Autodesk Inventor part; units mm, degrees
ref_plane "YZ Plane" through (0, 0, 0) normal (1, 0, 0) x (0, 1, 0)
ref_plane "XZ Plane" through (0, 0, 0) normal (0, 1, 0) x (-1, 0, 0)
ref_plane "XY Plane" through (0, 0, 0) normal (0, 0, 1) x (1, 0, 0)
sketch "スケッチ1" plane through (0, 0, 0) normal (0, 0, 1) x (1, 0, 0)
  line L0 (-6, 5) -> (6, 5)
  line L1 (6, 5) -> (6, -5)
  line L2 (6, -5) -> (-6, -5)
  line L3 (-6, -5) -> (-6, 5)
  point P0 (0, 0)
  point P1 (0, -5)
  point P2 (6, 0)
  dimension "d0" = 12
  dimension "d1" = 10
extrude "ギヤボックス" add sketch "スケッチ1" against normal blind 9
sketch "スケッチ2" plane through (0, 0, 0) normal (0, 0, 1) x (1, 0, 0)
  circle A0 centre (0, 0) radius 1.5
  line L0 (-1.118, 1) -> (1.118, 1)
  circle A1 centre (0, 0) radius 2
  dimension "d4" = 3
  dimension "d5" = 1
  dimension "d6" = 4
extrude "軸受け" add sketch "スケッチ2" along normal blind 0.7 contours A0 L0 | L0 A0 | A1
extrude "軸" add sketch "スケッチ2" along normal blind 10 contours A0 L0 picked at (0.0594, 0.1702)
sketch "スケッチ3" plane through (0, 0, -9) normal (0, 0, -1) x (-1, 0, 0)
  line L0 (6, 5) -> (-6, 5)
  line L1 (-6, -5) -> (6, -5)
  line L2 (-4, 5) -> (4, 5)
  line L3 (4, 5) -> (4, -5)
  line L4 (4, -5) -> (-4, -5)
  line L5 (-4, -5) -> (-4, 5)
  arc A0 (-4, 5) -> (-4, -5) centre (1.25, 0) ccw
  arc A1 (4, -5) -> (4, 5) centre (-1.25, 0) ccw
  line L6 (-6, 5) -> (-6, -5)
  line L7 (6, -5) -> (6, 5)
  line L8 (0, 7.0621) -> (0, -7.0621) construction
  line L9 (-6, 7.0625) -> (-6, -7.0625) construction
  line L10 (6, -7.0752) -> (6, 7.0489) construction
  point P0 (0, 0)
  point P1 (0, 5)
  point P2 (0, 0)
  point P3 (4, 5)
  point P4 (-4, -5)
  dimension "d11" = 8
  dimension "d15" = 12
extrude "モーター" add sketch "スケッチ3" along normal blind 15 contours L3 L1 L5 L0 | A1 L3 | L5 A0
sketch "スケッチ4" plane through (0, 0, -24) normal (0, 0, -1) x (-1, 0, 0)
  line L0 (-6.8, -5) -> (6.8, -5)
  line L1 (6.8, -5) -> (6.8, 5)
  line L2 (6.8, 5) -> (-6.8, 5)
  line L3 (-6.8, 5) -> (-6.8, -5)
  arc A0 (-6.8, -1.5) -> (-4.998, -5) centre (-2.5, -1.5) ccw
  arc A1 (4.998, -5) -> (6.8, -1.5) centre (2.5, -1.5) ccw
  line L4 (-4, -5) -> (4, -5)
  line L5 (0, 7.2835) -> (0, -7.2835) construction
  line L6 (-4.8, 5) -> (4.8, 5)
  line L7 (4.8, 5) -> (4.8, 8)
  line L8 (4.8, 8) -> (-4.8, 8)
  line L9 (-4.8, 8) -> (-4.8, 5)
  line L10 (4, 5) -> (-4, 5)
  point P0 (0, 0)
  point P1 (0, -5)
  point P2 (0, 0)
  point P3 (0, 8)
  dimension "d16" = 13.6
  dimension "d17" = 9.6
  dimension "d18" = 13
  dimension "d19" = 3.5
  dimension "d20" = 2.5
extrude "エンコーダ" add sketch "スケッチ4" along normal blind 8 contours A0 L3 L2 L1 A1 L0 | L9 L8 L7 L2
properties part number "MercuryN20"
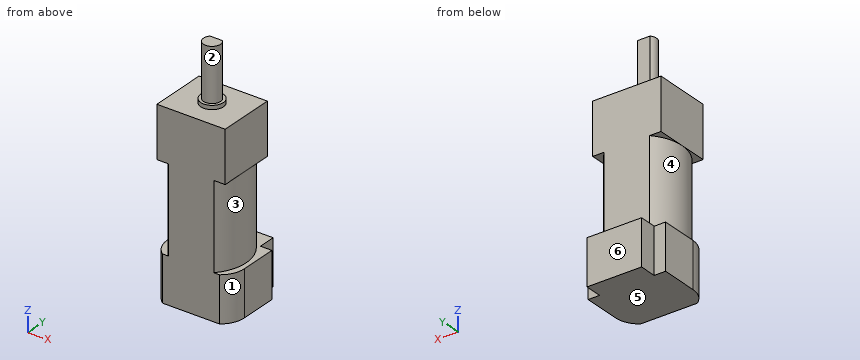
Can you work these out from the model? Positions are in its coordinate system, mm. Face numbers are marked on the shaded views. A direction names the side the tool comes from. Coordinates: 2 decimals unless noted, no trailing zeros. Write each loop counter-clockwise with the first axis right and the second up, starting at its lowest first coordinate (ties: lowest second). Pieces come first, ordered by that corner, then holes. Notation, with made-up numbers: M 17.5,-13.5 L 68.5,-13.5 A11 cw 68.5,-3.5 Z; hole C 49,-34.75 d10. An arc over 180 degrees is marked long. Use one line per item in the form item = value.
Q1. For P1, Ø2.5, axis at y = 6.5, z = -29, coming from the -X side; P2, Ø4.5, axis at y = 0.5, z = -4, coming from the -X side; P3, Ø5, axis at x = -2.5, y = 0, coming from the +Z side; P4, Ø0.7, axis at x = -0.5, z = 4.5, coming from the +Y side, each with a flat end and sliding along its axis, tell me the tip position at first contact or that it passes through.
Model answer:
P1 = -4.8
P2 = -6
P3 = 10
P4 = 1
Q2. If we section it at B-B (y = 6.75): Write out the boundary of the cut face in (x, z).
Model answer:
outline = M -4.8,-32 L 4.8,-32 L 4.8,-24 L -4.8,-24 Z
Q3. We'd pull the mould along Z, two halves only. Please class the marked faces 4, 5 and 6: +Z half, -Z half, draft (parallel to the pull), parting line (faces both ways), or undercut.
Model answer:
face_4 = undercut
face_5 = -Z half
face_6 = draft
Q4. If we section it at D-D (z = -18.5): Write out the boundary of the cut face in (x, y).
Model answer:
outline = M -4,-5 L 4,-5 A7.25 ccw 4,5 L -4,5 A7.25 ccw Z
Q5. I need wall thicknesses on line 1 along Z through (x, y) = (2.5, 2.25); line 2 along Y through (x, z) = (-1, -19.5); line 3 along Z through (x, y) = (-5.75, -2). Which ranges of each line are inside material? Lowest first, please. Write a range as from..to.
Model answer:
line_1 = -32..0
line_2 = -5..5
line_3 = -32..-24, -9..0
Q6. If we section it at A-A (x = 0): Write out the boundary of the cut face in (y, z).
Model answer:
outline = M -5,-32 L 8,-32 L 8,-24 L 5,-24 L 5,0 L 2,0 L 2,0.7 L 1,0.7 L 1,10 L -1.5,10 L -1.5,0.7 L -2,0.7 L -2,0 L -5,0 Z
Q7. For the marked faces 1, 2 and 3, which set-ups out of +Z, -Z, +X, -X, +Y, -Y let a thin tool reach every point of the face, with its end or its side?
Model answer:
face_1 = -Z, +X, -Y
face_2 = +Z
face_3 = +X
Q8. If we section it at C-C (x = 3.25): Write out the boundary of the cut face in (y, z).
Model answer:
outline = M -5,-32 L 8,-32 L 8,-24 L 5,-24 L 5,0 L -5,0 Z
